The model under review builds one solid part; all positions refer to its coordinate system, in mm. Face numbers are marked on the shaded views. Give positions to 0.01 mm unless a question says otherwise; leave off trailing zeros. Order: outer loops, then holes, each group sorted by start corner. A loop starts at its lowest first (then second) coordinate and runs counter-clockwise, first axis right, second up.
```python
from build123d import *

# Parameters (mm, degrees)
ESQUISSE1_W                                        = 93
ESQUISSE1_H                                        = 94
EXTRUSION1_DEPTH                                   = 8
CONG_1_R                                           = 6.3
CHAMBRAGE_POUR_VIS_T_TE_HEXAGONALE_M61_D           = 6.6
CHAMBRAGE_POUR_VIS_T_TE_HEXAGONALE_M61_CBORE_D     = 11
CHAMBRAGE_POUR_VIS_T_TE_HEXAGONALE_M61_CBORE_DEPTH = 6
ESQUISSE10_W                                       = 40
ESQUISSE10_H                                       = 25
ENL_V_MAT_EXTRU_1_DEPTH                            = 2
CONG_2_R                                           = 2


with BuildPart() as part:
    # Esquisse1 → Extrusion1 (new body)
    with BuildSketch(Plane.XY):
        Rectangle(ESQUISSE1_W, ESQUISSE1_H)
    extrude(amount=EXTRUSION1_DEPTH)

    # Congé1
    cong_1_edges = [part.edges().sort_by_distance(p)[0] for p in [
        (-46.5, 47, 4),
        (46.5, 47, 4),
        (46.5, -47, 4),
        (-46.5, -47, 4),
    ]]
    fillet(cong_1_edges, radius=CONG_1_R)

    # Chambrage pour vis à tête hexagonale M61 (through all)
    with Locations(Plane(origin=(0, 0, 0), x_dir=(-1, 0, 0), z_dir=(0, 0, -1))):
        with Locations((39.65, -40), (39.65, 40), (-39.65, 40), (-39.65, -40)):
            CounterBoreHole(CHAMBRAGE_POUR_VIS_T_TE_HEXAGONALE_M61_D / 2, CHAMBRAGE_POUR_VIS_T_TE_HEXAGONALE_M61_CBORE_D / 2, CHAMBRAGE_POUR_VIS_T_TE_HEXAGONALE_M61_CBORE_DEPTH)

    # Esquisse10 → Enlèv. mat.-Extru.1 (cut)
    with BuildSketch(Plane(origin=(0, 0, 0), x_dir=(-1, 0, 0), z_dir=(0, 0, -1))):
        with Locations((0, 22.804576525)):
            Rectangle(ESQUISSE10_W, ESQUISSE10_H)
    extrude(amount=-ENL_V_MAT_EXTRU_1_DEPTH, mode=Mode.SUBTRACT)

    # Congé2
    cong_2_edges = [part.edges().sort_by_distance(p)[0] for p in [
        (0, 35.304576525, 2),
        (-20, 22.804576525, 2),
        (0, 10.304576525, 2),
        (20, 22.804576525, 2),
    ]]
    fillet(cong_2_edges, radius=CONG_2_R - 0.0001)  # a hair under: the kernel refuses the full size


solid = part.part
```
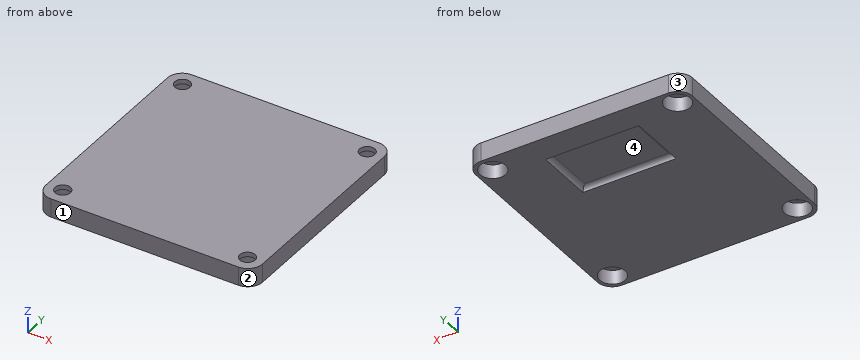
Item 1: Clearance check with flat-ended pins moving along their axes: pin 1 Ø8.5 at (x, y) = (-39.65, -40) entering from -Z; pin 2 Ø6.5 at (x, y) = (7.5, 23) entering from -Z; pin 3 Ø4 at (x, y) = (39.65, -40) entering from +Z. State where each tip first meets the part, or that it passes through.
Values found:
pin 1: stops at z = 6
pin 2: stops at z = 2
pin 3: passes through
Item 2: For line 1 (Y direction, x = 42.5, z = 5); line 2 (Y direction, x = 39.65, z = 7.1); line 3 (Y direction, x = -15.5, z = 1.5), list the stretches that pass through material, from the lowest coordinate up.
Values found:
line 1: y = -46.57 to -44.7, -35.3 to 35.3, 44.7 to 46.57
line 2: y = -47 to -43.3, -36.7 to 36.7, 43.3 to 47
line 3: y = -47 to 10.98, 34.63 to 47
Item 3: Draft analysis for pull direction X (two halves, no side actions). For the marked faces 1, 2, 3 and 4, state which applies: released by +X, released by -X, zero draft, split by the parting line, or undercut.
Values found:
face 1: zero draft
face 2: released by +X
face 3: released by -X
face 4: undercut
Item 4: Take a section at A-A (z = 4). Give the boundary of the cut face in (x, y), and give its area (3 significant figures).
Values found:
outline: (-46.5, -40.7) arc R6.3 ccw to (-40.2, -47) - (40.2, -47) arc R6.3 ccw to (46.5, -40.7) - (46.5, 40.7) arc R6.3 ccw to (40.2, 47) - (-40.2, 47) arc R6.3 ccw to (-46.5, 40.7) - close; hole circle Ø11 at (-39.65, -40); hole circle Ø11 at (-39.65, 40); hole circle Ø11 at (39.65, -40); hole circle Ø11 at (39.65, 40)
area: 8,330 mm2
